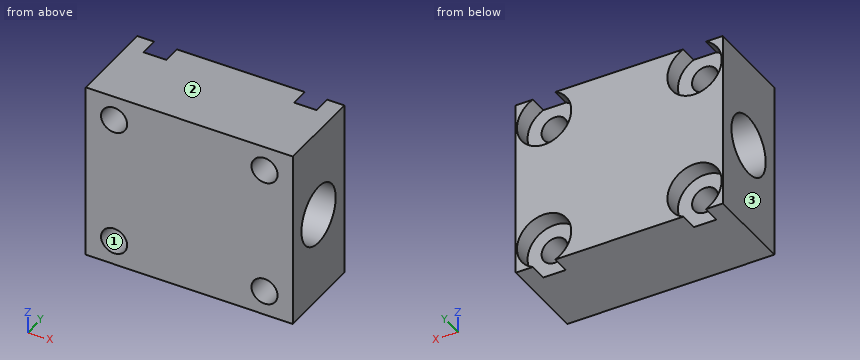
from build123d import *

# Parameters (mm, degrees)
SKETCH1_W                                        = 42
SKETCH1_H                                        = 36
BOSS_EXTRUDE1_DEPTH                              = 18
CBORE_FOR_M5_PAN_HEAD_MACHINE_SCREW3_D           = 5.3
CBORE_FOR_M5_PAN_HEAD_MACHINE_SCREW3_CBORE_D     = 11
CBORE_FOR_M5_PAN_HEAD_MACHINE_SCREW3_CBORE_DEPTH = 3.7
SKETCH7_R                                        = 6
CUT_EXTRUDE1_DEPTH                               = 50.112116631


with BuildPart() as part:
    # Sketch1 → Boss-Extrude1 (new body)
    with BuildSketch(Plane(origin=(0, 0, 0), x_dir=(1, 0, 0), z_dir=(0, 1, 0))):
        Rectangle(SKETCH1_W, SKETCH1_H)
    extrude(amount=BOSS_EXTRUDE1_DEPTH)

    # CBORE for M5 Pan Head Machine Screw3 (through all)
    with Locations(Plane(origin=(-6.549083899, 18, -3.689624732), x_dir=(-1, 0, 0), z_dir=(0, 1, 0))):
        with Locations((8.700916101, 16.689624732), (-21.799083899, 16.689624732), (-21.799083899, -9.310375268), (8.700916101, -9.310375268)):
            CounterBoreHole(CBORE_FOR_M5_PAN_HEAD_MACHINE_SCREW3_D / 2, CBORE_FOR_M5_PAN_HEAD_MACHINE_SCREW3_CBORE_D / 2, CBORE_FOR_M5_PAN_HEAD_MACHINE_SCREW3_CBORE_DEPTH)

    # Sketch7 → Cut-Extrude1 (cut, through all)
    with BuildSketch(Plane(origin=(21, 0, 0), x_dir=(0, 0, -1), z_dir=(1, 0, 0))):
        with Locations((0, 9)):
            Circle(SKETCH7_R)
    extrude(amount=-CUT_EXTRUDE1_DEPTH, mode=Mode.SUBTRACT)


solid = part.part
Geometry check sheet. Reference: the model listing, model coordinates, mm. Face numbers are marked on the shaded views. Coordinates: 2 decimals unless noted, no trailing zeros. Write each loop counter-clockwise with the first axis right and the second up, starting at its lowest first coordinate (ties: lowest second). Pieces come first, ordered by that corner, then holes. Notation, with made-up numbers: (60.5, 0.25) -> (102.5, 0.25) arc R20 cw to (102.5, 35.25) -> close; hole circle Ø1 at (58.25, 27). An arc over 180 degrees is marked (long way). One line per question, with ' | ' between items.
1. Cross-section at A-A on z = -13. Record the cut outline in (x, y), and give its area (3 significant figures).
Answers:
outline: (-21, 0) -> (-17.9, 0) -> (-17.9, 14.3) -> (-20.75, 14.3) -> (-20.75, 18) -> (-21, 18) -> close; (-12.6, 0) -> (12.6, 0) -> (12.6, 14.3) -> (9.75, 14.3) -> (9.75, 18) -> (-9.75, 18) -> (-9.75, 14.3) -> (-12.6, 14.3) -> close; (17.9, 0) -> (21, 0) -> (21, 18) -> (20.75, 18) -> (20.75, 14.3) -> (17.9, 14.3) -> close | area: 523 mm²
2. Cross-section at B-B on x = 15.25. Record the cut outline in (y, z), and give its area (3 significant figures).
Answers:
outline: (0, -18) -> (14.3, -18) -> (14.3, -15.65) -> (0, -15.65) -> close; (0, -10.35) -> (14.3, -10.35) -> (14.3, -7.5) -> (18, -7.5) -> (18, 7.5) -> (14.3, 7.5) -> (14.3, 10.35) -> (0, 10.35) -> close; (0, 15.65) -> (14.3, 15.65) -> (14.3, 18) -> (0, 18) -> close; hole circle Ø12 at (9, 0) | area: 306 mm²
3. Draft check along X on the marked faces 1, 2 and 3. Enter one of: +X half, -X half, draft (parallel to the pull), parting line (faces both ways), or undercut.
Answers:
face 1: undercut | face 2: draft | face 3: -X half
4. Cross-section at D-D on z = 0. Record the cut outline in (x, y).
Answers:
outline: (-21, 0) -> (21, 0) -> (21, 3) -> (-21, 3) -> close; (-21, 15) -> (21, 15) -> (21, 18) -> (-21, 18) -> close
5. Depth check by flat-ended pin: pin 1 Ø3 at (x, z) = (15, -11) entering from +Y; pin 2 Ø4 at (x, z) = (15.25, -13) entering from +Y. Enter the tip coordinate at first touch or a pass-through.
Answers:
pin 1: stops at y = 14.3 | pin 2: passes through
6. Cross-section at C-C on y = 10.75. Record the cut outline in (x, z), and give its area (3 significant figures).
Answers:
outline: (-21, -18) -> (21, -18) -> (21, -5.74) -> (-21, -5.74) -> close; (-21, 5.74) -> (21, 5.74) -> (21, 18) -> (-21, 18) -> close; hole circle Ø5.3 at (-15.25, -13); hole circle Ø5.3 at (-15.25, 13); hole circle Ø5.3 at (15.25, -13); hole circle Ø5.3 at (15.25, 13) | area: 942 mm²
7. Thickness scan on probe 1 along X at (y, z) = (15.1, -13); probe 2 along Z at (x, y) = (-15.25, 10.75); probe 3 along X at (y, z) = (4.25, 12.5). Record the ranges inside material, lowest first. Write a range as from..to.
Answers:
probe 1: x = -21..-20.75, -9.75..9.75, 20.75..21 | probe 2: z = -18..-15.65, -10.35..-5.74, 5.74..10.35, 15.65..18 | probe 3: x = -21..-17.85, -12.65..12.65, 17.85..21
